```python
from build123d import *

# Parameters (mm, degrees)
SKETCH1_W           = 126
SKETCH1_H           = 126
BOSS_EXTRUDE1_DEPTH = 5
SKETCH3_R           = 12.5
BOSS_EXTRUDE2_DEPTH = 7.5
SKETCH4_R           = 3.45
CUT_EXTRUDE1_DEPTH  = 11.5
SKETCH6_R           = 3
CUT_EXTRUDE2_DEPTH  = 179.628805068
CHAMFER1_SIZE       = 10
CHAMFER1_SIZE_2     = 7.26542528


with BuildPart() as part:
    # Sketch1 → Boss-Extrude1 (new body)
    with BuildSketch(Plane(origin=(0, 0, 0), x_dir=(1, 0, 0), z_dir=(0, 1, 0))):
        with Locations((63, 63)):
            Rectangle(SKETCH1_W, SKETCH1_H)
    extrude(amount=BOSS_EXTRUDE1_DEPTH)

    # Sketch3 → Boss-Extrude2 (add)
    with BuildSketch(Plane(origin=(0, 5, 0), x_dir=(1, 0, 0), z_dir=(0, 1, 0))):
        with Locations(Location((108.6, 108.6, 0), (0, 0, 90))):
            Circle(SKETCH3_R)
    extrude(amount=BOSS_EXTRUDE2_DEPTH)

    # Sketch4 → Cut-Extrude1 (cut)
    with BuildSketch(Plane.XZ):
        with Locations(Location((108.6, -108.6, 0), (0, 0, 270))):
            Circle(SKETCH4_R)
    extrude(amount=-CUT_EXTRUDE1_DEPTH, mode=Mode.SUBTRACT)

    # Sketch6 → Cut-Extrude2 (cut, through all)
    with BuildSketch(Plane(origin=(0, 12.5, 0), x_dir=(1, 0, 0), z_dir=(0, 1, 0))):
        with Locations(Location((108.6, 108.6, 0), (0, 0, 270))):
            Circle(SKETCH6_R)
    extrude(amount=-CUT_EXTRUDE2_DEPTH, mode=Mode.SUBTRACT)

    # Chamfer1
    # the kernel refuses this chamfer: 10, 7.26542528 mm, written as the material it takes off along each edge
    with BuildSketch(Plane(origin=(108.6, 12.5, -108.6), x_dir=(0, 0, -1), z_dir=(1, 0, 0))) as chamfer1_piece_1_section:
        Polygon((12.5, -CHAMFER1_SIZE), (12.5 - CHAMFER1_SIZE_2, 0), (12.5, 0), align=None)
    chamfer1_piece_1 = revolve(axis=Axis((108.6, 12.5, -108.6), (0, 1, 0)), mode=Mode.PRIVATE)
    chamfer1_piece_1 = split(chamfer1_piece_1, bisect_by=Plane(origin=(108.6, 5, -100.650989912), z_dir=(0, 1, 0)), keep=Keep.TOP, mode=Mode.PRIVATE)
    add(chamfer1_piece_1, mode=Mode.SUBTRACT)


solid = part.part
```
Verification items for the finished model (mm, model axes). Coordinates: 2 decimals unless noted, no trailing zeros. Order: outer loops, then holes, each group sorted by start corner. A loop starts at its lowest first (then second) coordinate and runs counter-clockwise, first axis right, second up. Notation, with made-up numbers: (26.25, 86) - (84.25, 86) arc R23 cw to (84.25, 109) - close; hole circle Ø7 at (88.25, 61.25). An arc over 180 degrees is marked (long way). Return JSON: item names as keys, results as strings.
(1) Thickness scan on line 1 along Z through (x, y) = (109, 4); line 2 along X through (y, z) = (2.5, -108.6); line 3 along Y through (x, z) = (63, -34.5). Record the ranges inside material, lowest first.
Filled sheet:
{"line 1": "z = -126 to -112.03, -105.17 to 0", "line 2": "x = 0 to 105.15, 112.05 to 126", "line 3": "y = 0 to 5"}
(2) Go/stop test with a flat-tipped pin: pin 1 (2 mm diameter, centred on x = 73.5, z = -32, fed in from +Y). Record where the tip stops, or that it passes through.
Filled sheet:
{"pin 1": "stops at y = 5"}
(3) Mould release check, pull along X, two halves, no side actions. Record for faces 1 (the flat face through (62, 2, 0)), 2 (the flat face through (0, 2, -62)), 3 (the cylindrical face through (111.51, 5.67, -110.45)), 4 (the cylindrical face through (105.67, 12.01, -109.25)): pulls with the +X half, pulls with the -X half, needs draft (parallel to the pull), parting line crosses it, or undercut.
Filled sheet:
{"face 1": "needs draft", "face 2": "pulls with the -X half", "face 3": "undercut", "face 4": "undercut"}
(4) Section check D-D, the plane x = 87. Record the cut outline in (y, z), and give its area (3 significant figures).
Filled sheet:
{"outline": "(0, -126) - (5, -126) - (5, 0) - (0, 0) - close", "area": "630 mm^2"}
(5) Section check C-C, the plane y = 6.5. Record the cut outline in (x, z), and give its area (3 significant figures).
Filled sheet:
{"outline": "circle Ø19.19 at (108.6, -108.6); hole circle Ø6.9 at (108.6, -108.6)", "area": "252 mm^2"}
(6) Section check B-B, the plane z = -108.6. Record the cut outline in (x, y), and give its area (3 significant figures).
Filled sheet:
{"outline": "(0, 0) - (105.15, 0) - (105.15, 11.5) - (105.6, 11.5) - (105.6, 12.5) - (103.37, 12.5) - (97.92, 5) - (0, 5) - close; (111.6, 11.5) - (112.05, 11.5) - (112.05, 0) - (126, 0) - (126, 5) - (119.28, 5) - (113.83, 12.5) - (111.6, 12.5) - close", "area": "664 mm^2"}
(7) Section check A-A, the plane x = 108.6. Record the cut outline in (y, z), and give its area (3 significant figures).
Filled sheet:
{"outline": "(0, -126) - (5, -126) - (5, -119.28) - (12.5, -113.83) - (12.5, -111.6) - (11.5, -111.6) - (11.5, -112.05) - (0, -112.05) - close; (0, -105.15) - (11.5, -105.15) - (11.5, -105.6) - (12.5, -105.6) - (12.5, -103.37) - (5, -97.92) - (5, 0) - (0, 0) - close", "area": "664 mm^2"}
